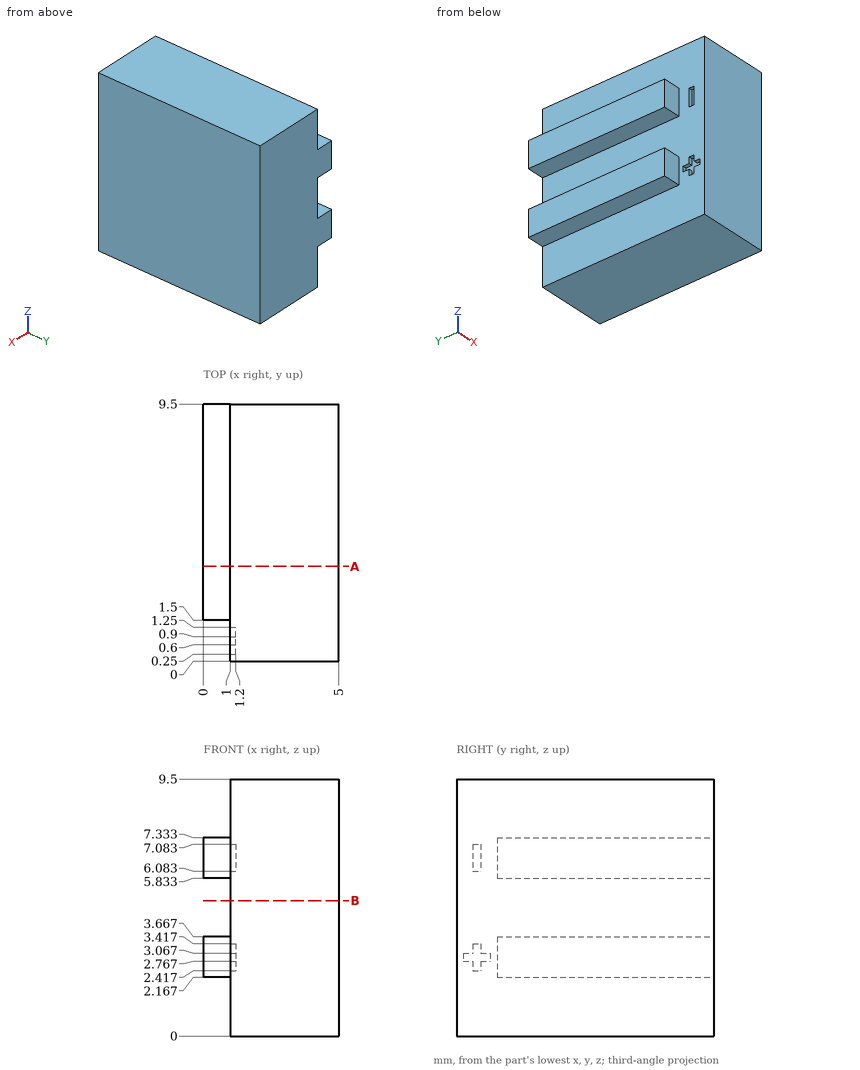
Input: dimensioned drawing with shaded views. Units: mm. Origin: part minimum x, y, z. Give positions to 0.01 mm unless a question says otherwise; leave off trailing zeros. Write each loop counter-clockwise with the first axis right and the second up, starting at its lowest first coordinate (ties: lowest second). Pieces come first, ordered by that corner, then holes. Notation, with made-up numbers: (20, 28.25) -> (37, 28.25) arc R31 cw to (37, 52.25) -> close; hole circle Ø7 at (76, 54). An arc over 180 degrees is marked (long way). Return JSON: item names as keys, results as strings. Group by question number.
1. Section B-B, the plane z = 5. Output: boundary loops of the cut face in (x, y), then the cut area to 3 significant figures.
2. Pin query (flat end, axial travel): pin 1 Ø0.5 at (x, y) = (0.5, 6) entering from +Z. Return the tip coordinate at first contact, or that it passes through.
3. Section A-A, the plane y = 3.5. Output: boundary loops of the cut face in (x, z), then the cut area to 3 significant figures.
4. Material intervals for line 1 (Z direction, x = 0.4, y = 5); line 2 (Y direction, x = 1.15, z = 2.5); line 3 (X direction, y = 9.25, z = 1), sorted ascending. Write a range as from..to.
Determined:
{
 "1": {"outline": "(1, 0) -> (5, 0) -> (5, 9.5) -> (1, 9.5) -> close", "area": "38.0 mm2"},
 "2": {"pin 1": "stops at z = 7.33"},
 "3": {"outline": "(0, 2.17) -> (1, 2.17) -> (1, 0) -> (5, 0) -> (5, 9.5) -> (1, 9.5) -> (1, 7.33) -> (0, 7.33) -> (0, 5.83) -> (1, 5.83) -> (1, 3.67) -> (0, 3.67) -> close", "area": "41.0 mm2"},
 "4": {"line 1": "z = 2.17..3.67, 5.83..7.33", "line 2": "y = 0..0.6, 0.9..9.5", "line 3": "x = 1..5"}
}
